Read the model definition and answer for the solid it produces. Units are mm, in the model's axes. Coordinates: 2 decimals unless noted, no trailing zeros. Loops run counter-clockwise (first coordinate to the right, second up) from the corner with the lowest first, then second, coordinate; pieces in that order, holes last. Notation, with made-up numbers: (-22, 9) -> (18, 9) arc R25 cw to (18, 28) -> close; hole circle Ø1 at (-12, 7). An arc over 180 degrees is marked (long way). Answer in a Markdown table with one row per item.
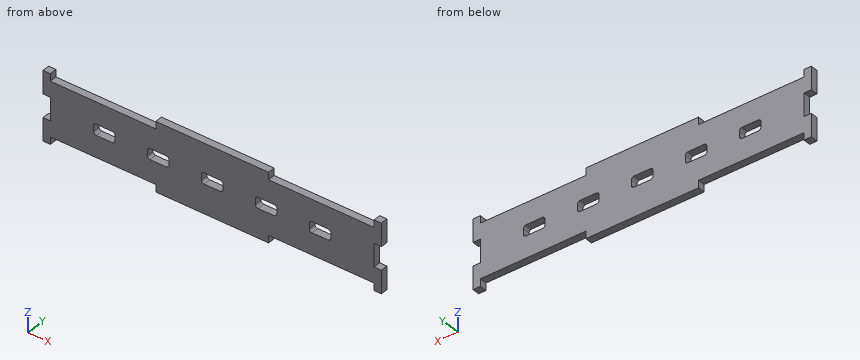
```python
from build123d import *

# Parameters (mm, degrees)
BOSS_EXTRUDE1_DEPTH = 2.7


with BuildPart() as part:
    # Sketch1 → Boss-Extrude1 (new body)
    with BuildSketch(Plane(origin=(0, 0, 0), x_dir=(1, 0, 0), z_dir=(0, 1, 0))):
        Polygon((-62.7, 12.7), (-60, 12.7), (-60, 10), (-20.9, 10), (-20.9, 12.7), (20.9, 12.7), (20.9, 10), (60, 10), (60, 12.7), (62.7, 12.7), (62.7, 4.233333333), (60, 4.233333333), (60, -4.233333333), (62.7, -4.233333333), (62.7, -12.7), (60, -12.7), (60, -10), (20.9, -10), (20.9, -12.7), (-20.9, -12.7), (-20.9, -10), (-60, -10), (-60, -12.7), (-62.7, -12.7), (-62.7, -4.233333333), (-60, -4.233333333), (-60, 4.233333333), (-62.7, 4.233333333), align=None)
        with BuildLine():
            Line((-37, 2), (-43, 2))
            ThreePointArc((-43, 2), (-43.707106781, 1.707106781), (-44, 1))
            Line((-44, 1), (-44, -1))
            ThreePointArc((-44, -1), (-43.707106781, -1.707106781), (-43, -2))
            Line((-43, -2), (-37, -2))
            ThreePointArc((-37, -2), (-36.292893219, -1.707106781), (-36, -1))
            Line((-36, -1), (-36, 1))
            ThreePointArc((-36, 1), (-36.292893219, 1.707106781), (-37, 2))
        make_face(mode=Mode.SUBTRACT)
        with BuildLine():
            Line((-23, 2), (-17, 2))
            ThreePointArc((-17, 2), (-16.292893219, 1.707106781), (-16, 1))
            Line((-16, 1), (-16, -1))
            ThreePointArc((-16, -1), (-16.292893219, -1.707106781), (-17, -2))
            Line((-17, -2), (-23, -2))
            ThreePointArc((-23, -2), (-23.707106781, -1.707106781), (-24, -1))
            Line((-24, -1), (-24, 1))
            ThreePointArc((-24, 1), (-23.707106781, 1.707106781), (-23, 2))
        make_face(mode=Mode.SUBTRACT)
        with BuildLine():
            Line((-3, 2), (3, 2))
            ThreePointArc((3, 2), (3.707106781, 1.707106781), (4, 1))
            Line((4, 1), (4, -1))
            ThreePointArc((4, -1), (3.707106781, -1.707106781), (3, -2))
            Line((3, -2), (-3, -2))
            ThreePointArc((-3, -2), (-3.707106781, -1.707106781), (-4, -1))
            Line((-4, -1), (-4, 1))
            ThreePointArc((-4, 1), (-3.707106781, 1.707106781), (-3, 2))
        make_face(mode=Mode.SUBTRACT)
        with BuildLine():
            Line((17, 2), (23, 2))
            ThreePointArc((23, 2), (23.707106781, 1.707106781), (24, 1))
            Line((24, 1), (24, -1))
            ThreePointArc((24, -1), (23.707106781, -1.707106781), (23, -2))
            Line((23, -2), (17, -2))
            ThreePointArc((17, -2), (16.292893219, -1.707106781), (16, -1))
            Line((16, -1), (16, 1))
            ThreePointArc((16, 1), (16.292893219, 1.707106781), (17, 2))
        make_face(mode=Mode.SUBTRACT)
        with BuildLine():
            Line((37, 2), (43, 2))
            ThreePointArc((43, 2), (43.707106781, 1.707106781), (44, 1))
            Line((44, 1), (44, -1))
            ThreePointArc((44, -1), (43.707106781, -1.707106781), (43, -2))
            Line((43, -2), (37, -2))
            ThreePointArc((37, -2), (36.292893219, -1.707106781), (36, -1))
            Line((36, -1), (36, 1))
            ThreePointArc((36, 1), (36.292893219, 1.707106781), (37, 2))
        make_face(mode=Mode.SUBTRACT)
    extrude(amount=BOSS_EXTRUDE1_DEPTH)


solid = part.part
```
1. A cutting plane is placed at A-A on x = -19. Give the vertices of the cut face in (y, z).
A:
| item | result |
|---|---|
| outline | (0, -12.7) -> (2.7, -12.7) -> (2.7, -2) -> (0, -2) -> close; (0, 2) -> (2.7, 2) -> (2.7, 12.7) -> (0, 12.7) -> close |
2. A cutting plane is placed at B-B on y = 1.2. Count the separate pieces of the cut face and the enclosed holes in it, and give its area (3 significant figures).
A:
| item | result |
|---|---|
| separate pieces | 1 |
| enclosed holes | 5 |
| area | 2,560 mm2 |
3. Find the intervals of material crossed by probe 1 along X at (y, z) = (2.5, -0.25); probe 2 along X at (y, z) = (1.6, 10.5); probe 3 along Z at (x, y) = (-20.5, 2.2), in increasing order.
A:
| item | result |
|---|---|
| probe 1 | x = -60 to -44, -36 to -24, -16 to -4, 4 to 16, 24 to 36, 44 to 60 |
| probe 2 | x = -62.7 to -60, -20.9 to 20.9, 60 to 62.7 |
| probe 3 | z = -12.7 to -2, 2 to 12.7 |
4. Given pin 1 Ø1.4 at (y, z) = (1, -2) entering from -X; pin 2 Ø2 at (x, z) = (-37, 8) entering from -Y, each flat-ended and moving along its own axis, determine where each tip first touches the part or whether it passes through.
A:
| item | result |
|---|---|
| pin 1 | stops at x = -60 |
| pin 2 | stops at y = 0 |
